```python
from build123d import *

# Parameters (mm, degrees)
ESBO_O1_W                = 20
ESBO_O1_H                = 3
ESBO_O1_W_2              = 3
ESBO_O1_H_2              = 20
RESSALTO_EXTRUS_O1_DEPTH = 3


with BuildPart() as part:
    # Esboço1 → Ressalto-extrusão1 (new body)
    with BuildSketch(Plane.XY):
        Polygon((208.901159766, 291.53692045), (233.901159766, 291.53692045), (233.901159766, 306.53692045), (188.901159766, 306.53692045), (188.901159766, 266.53692045), (158.901159766, 266.53692045), (158.901159766, 265.03692045), (138.901159766, 265.03692045), (138.901159766, 266.53692045), (98.901159766, 266.53692045), (98.901159766, 265.03692045), (78.901159766, 265.03692045), (78.901159766, 266.53692045), (48.901159766, 266.53692045), (48.901159766, 306.53692045), (3.901159766, 306.53692045), (3.901159766, 291.53692045), (28.901159766, 291.53692045), (28.901159766, 266.53692045), (-31.098840234, 266.53692045), (-31.098840234, -33.46307955), (268.901159766, -33.46307955), (268.901159766, 26.53692045), (293.901159766, 26.53692045), (293.901159766, 1.53692045), (308.901159766, 1.53692045), (308.901159766, 46.53692045), (268.901159766, 46.53692045), (268.901159766, 76.53692045), (267.401159766, 76.53692045), (267.401159766, 96.53692045), (268.901159766, 96.53692045), (268.901159766, 136.53692045), (267.401159766, 136.53692045), (267.401159766, 156.53692045), (268.901159766, 156.53692045), (268.901159766, 186.53692045), (308.901159766, 186.53692045), (308.901159766, 231.53692045), (293.901159766, 231.53692045), (293.901159766, 206.53692045), (268.901159766, 206.53692045), (268.901159766, 266.53692045), (208.901159766, 266.53692045), align=None)
        with Locations((88.901159766, -29.46307955)):
            Rectangle(ESBO_O1_W, ESBO_O1_H, mode=Mode.SUBTRACT)
        with Locations((148.901159766, -29.46307955)):
            Rectangle(ESBO_O1_W, ESBO_O1_H, mode=Mode.SUBTRACT)
        with Locations((-27.098840234, 146.53692045)):
            Rectangle(ESBO_O1_W_2, ESBO_O1_H_2, mode=Mode.SUBTRACT)
        with Locations((-27.098840234, 86.53692045)):
            Rectangle(ESBO_O1_W_2, ESBO_O1_H_2, mode=Mode.SUBTRACT)
    extrude(amount=RESSALTO_EXTRUS_O1_DEPTH)


solid = part.part
```
Model file for the job. Use its own axes, mm. Round coordinates to 2 decimals unless told otherwise and drop trailing zeros. Write each loop counter-clockwise with the first axis right and the second up, starting at its lowest first coordinate (ties: lowest second). Pieces come first, ordered by that corner, then holes. Notation, with made-up numbers: (51, 12) - (83, 12) arc R21 ccw to (83, 16) - close; hole circle Ø6 at (-10, 64). An arc over 180 degrees is marked (long way). One line per item, written item: value.
(1) Drop flat-ended pins along their axis: P1, Ø1.5, axis at y = 149.5, z = 2, coming from the +X side; P2, Ø8, axis at x = 195, y = 72.5, coming from the -Z side; P3, Ø0.9, axis at y = 281.5, z = 1, coming from the +X side; P4, Ø0.9, axis at x = 151, z = 1.5, coming from the +Y side. Give the stop position or say it passes through.
Values follow:
P1: stops at x = 267.4
P2: stops at z = 0
P3: stops at x = 208.9
P4: stops at y = 265.04
(2) Wall check: probe 1 along Y at (x, z) = (279, 0.8); probe 2 along Y at (x, z) = (139, 0.95); probe 3 along X at (y, z) = (24.5, 1.8). Give the ranges that are in metal, low to high.
Values follow:
probe 1: y = 26.54 to 46.54, 186.54 to 206.54
probe 2: y = -33.46 to -30.96, -27.96 to 265.04
probe 3: x = -31.1 to 268.9, 293.9 to 308.9
(3) Cut at D-D, the plane y = 244. Give the cut face in (x, z).
Values follow:
outline: (-31.1, 0) - (268.9, 0) - (268.9, 3) - (-31.1, 3) - close
(4) Cut at A-A, the plane y = 12. Give the cut face in (x, z).
Values follow:
outline: (-31.1, 0) - (268.9, 0) - (268.9, 3) - (-31.1, 3) - close; (293.9, 0) - (308.9, 0) - (308.9, 3) - (293.9, 3) - close
(5) Cut at B-B, the plane x = 22. Give the cut face in (y, z).
Values follow:
outline: (-33.46, 0) - (266.54, 0) - (266.54, 3) - (-33.46, 3) - close; (291.54, 0) - (306.54, 0) - (306.54, 3) - (291.54, 3) - close
(6) Cut at C-C, the plane z = 0.75. Give the number of separate pieces and of enclosed holes in the cut face, plus the area to 3 significant figures.
Values follow:
separate pieces: 1
enclosed holes: 4
area: 94,300 mm²
